Verification items for the finished model (mm, model axes). Face numbers are marked on the shaded views. Round coordinates to 2 decimals unless told otherwise and drop trailing zeros. Order: outer loops, then holes, each group sorted by start corner. A loop starts at its lowest first (then second) coordinate and runs counter-clockwise, first axis right, second up. Notation, with made-up numbers: (72.25, 3.5) -> (109.25, 3.5) arc R22 ccw to (109.25, 30.5) -> close; hole circle Ø4 at (63, -6). An arc over 180 degrees is marked (long way). Return JSON: item names as keys, results as strings. Group by question number.
1) Scan lines: L1, parallel to Y at x = 0, z = -3; L2, parallel to Z at x = -14, y = 5; L3, parallel to Z at x = -0.5, y = -5.5. Record each from-to range of solid material in increasing order.
2) Depth check by flat-ended pin: pin 1 (10 mm diameter, centred on y = -1, z = -9.5, fed in from +X); pin 2 (1.6 mm diameter, centred on x = 0, y = -13.5, fed in from +Z); pin 3 (2.5 mm diameter, centred on x = -13.5, y = -0.5, fed in from +Z). Enter the tip coordinate at first touch or a pass-through.
3) Draft check along X on the marked faces 1 and 2. Enter one of: pulls with the +X half, pulls with the -X half, needs draft (parallel to the pull), parting line crosses it, or undercut.
4) Section check A-A on x = 0. Enter the section's corners in (y, z).
5) Section check C-C on z = 4.5. Enter the section's corners in (x, y).
6) Section check D-D on x = -13. Enter the section's corners in (y, z).
Autodesk Inventor part; units mm, degrees
ref_plane "YZ Plane" through (0, 0, 0) normal (1, 0, 0) x (0, 1, 0)
ref_plane "XZ Plane" through (0, 0, 0) normal (0, 1, 0) x (-1, 0, 0)
ref_plane "XY Plane" through (0, 0, 0) normal (0, 0, 1) x (1, 0, 0)
sketch "スケッチ1" plane through (0, 0, 0) normal (0, 0, 1) x (1, 0, 0)
  circle A0 centre (0, 0) radius 16
  dimension "d0" = 32
extrude "押し出し1" add sketch "スケッチ1" against normal blind 26
sketch "スケッチ2" plane through (0, 0, -26) normal (0, 0, -1) x (-1, 0, 0)
  circle A0 centre (0, 0) radius 17.5
  dimension "d3" = 35
extrude "押し出し2" add sketch "スケッチ2" along normal blind 71
sketch "スケッチ3" plane through (0, 0, 0) normal (0, 0, 1) x (1, 0, 0)
  circle A0 centre (0, 13) radius 1.6
  point P0 (0, 0)
  dimension "d6" = 3.2
  dimension "d7" = 13
extrude "押し出し3" cut sketch "スケッチ3" against normal blind 5
pattern_circular "円形状パターン1" count 4 over 360 about axis through (0, 0, -10) along (0, 0, 1) of "押し出し3"
sketch "スケッチ4" plane through (0, 0, 0) normal (0, 0, 1) x (1, 0, 0)
  circle A0 centre (0, 0) radius 9.5
  dimension "d13" = 19
extrude "押し出し4" add sketch "スケッチ4" along normal blind 2
sketch "スケッチ5" plane through (0, 0, 2) normal (0, 0, 1) x (1, 0, 0)
  circle A0 centre (0, 0) radius 3
  dimension "d16" = 6
extrude "押し出し5" add sketch "スケッチ5" along normal blind 19
properties part number "motor" material "アルミニウム 6061"
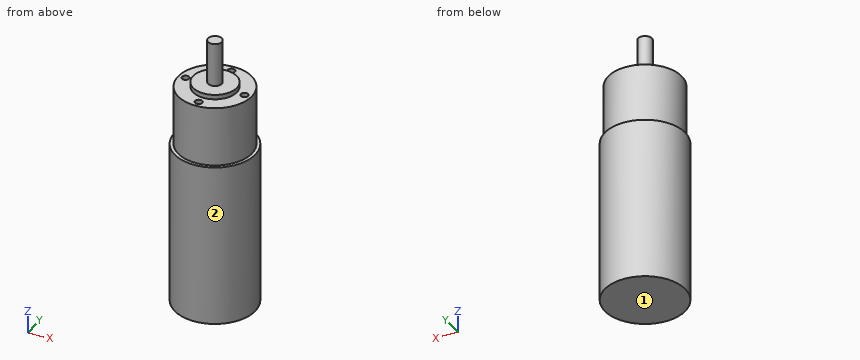
Check result:
{
 "1": {"L1": "-16 to -14.6, -11.4 to 11.4, 14.6 to 16", "L2": "-97 to 0", "L3": "-97 to 2"},
 "2": {"pin 1": "x = 16", "pin 2": "z = -5", "pin 3": "z = 0"},
 "3": {"face 1": "needs draft", "face 2": "parting line crosses it"},
 "4": {"outline": "(-17.5, -97) -> (17.5, -97) -> (17.5, -26) -> (16, -26) -> (16, 0) -> (14.6, 0) -> (14.6, -5) -> (11.4, -5) -> (11.4, 0) -> (9.5, 0) -> (9.5, 2) -> (3, 2) -> (3, 21) -> (-3, 21) -> (-3, 2) -> (-9.5, 2) -> (-9.5, 0) -> (-11.4, 0) -> (-11.4, -5) -> (-14.6, -5) -> (-14.6, 0) -> (-16, 0) -> (-16, -26) -> (-17.5, -26) -> close"},
 "5": {"outline": "circle Ø6 at (0, 0)"},
 "6": {"outline": "(-11.72, -97) -> (11.72, -97) -> (11.72, -26) -> (9.33, -26) -> (9.33, 0) -> (1.6, 0) -> (1.6, -5) -> (-1.6, -5) -> (-1.6, 0) -> (-9.33, 0) -> (-9.33, -26) -> (-11.72, -26) -> close"}
}
